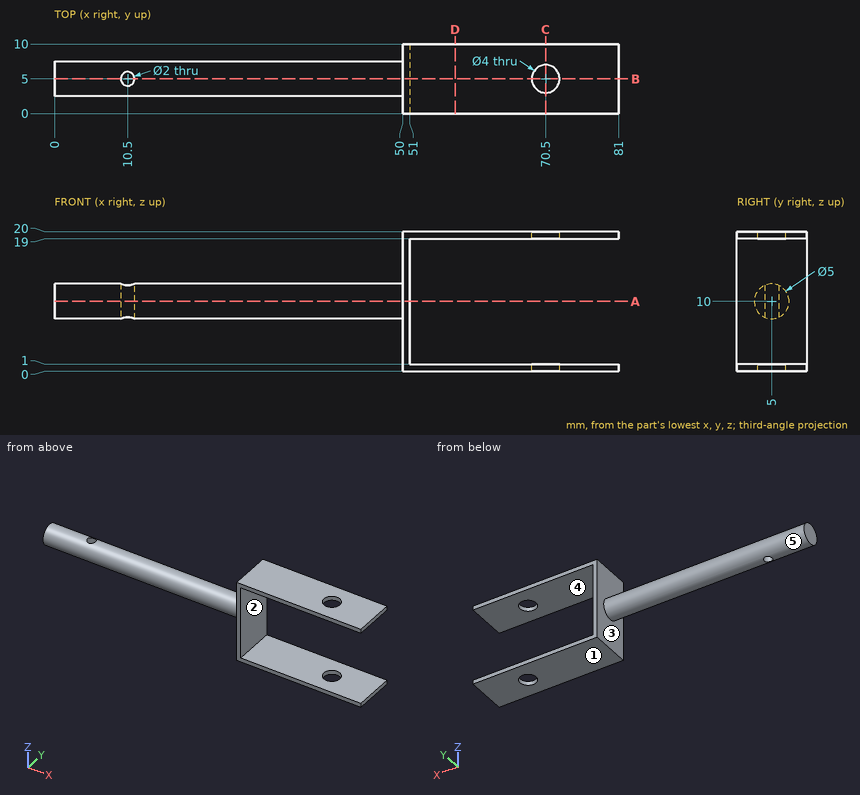
Input: dimensioned drawing with shaded views. Units: mm. Origin: part minimum x, y, z. A direction names the side the tool comes from. Give positions to 0.01 mm unless a question says otherwise; leave off trailing zeros. Order: outer loops, then holes, each group sorted by start corner. A loop starts at its lowest first (then second) coordinate and runs counter-clockwise, first axis right, second up. Notation, with made-up numbers: (55, 27.5) -> (98, 27.5) arc R25 cw to (98, 48.5) -> close; hole circle Ø9 at (-26, 39.25). An arc over 180 degrees is marked (long way). Answer as a JSON object with one key per item and string values.
Q1. First-contact query: pin 1 (1.6 mm diameter, centred on x = 10.5, y = 5, fed in from +Z); pin 2 (3 mm diameter, centred on x = 32.5, y = 6, fed in from +Z); pin 3 (1.5 mm diameter, centred on x = 44, y = 6, fed in from -Z); pin 4 (3 mm diameter, centred on y = 6.5, z = 12, fed in from +X). Flat tips, straight axial feed; report the tip coordinate or a pass-through.
Entries:
{"pin 1": "passes through", "pin 2": "stops at z = 12.5", "pin 3": "stops at z = 7.51", "pin 4": "stops at x = 51"}
Q2. Section D-D (x = 57.5). Output: boundary loops of the cut face in (y, z), plus the area to 3 significant figures.
Entries:
{"outline": "(0, 0) -> (10, 0) -> (10, 1) -> (0, 1) -> close; (0, 19) -> (10, 19) -> (10, 20) -> (0, 20) -> close", "area": "20.0 mm^2"}
Q3. Material intervals for probe 1 along X at (y, z) = (5, 8.6); probe 2 along X at (y, z) = (5, 19.75); probe 3 along Z at (x, y) = (69.5, 1.5), sorted ascending.
Entries:
{"probe 1": "x = 0 to 9.5, 11.5 to 51", "probe 2": "x = 50 to 68.5, 72.5 to 81", "probe 3": "z = 0 to 1, 19 to 20"}
Q4. Section A-A (z = 10). Output: boundary loops of the cut face in (x, y), plus the area to 3 significant figures.
Entries:
{"outline": "(0, 2.5) -> (50, 2.5) -> (50, 0) -> (51, 0) -> (51, 10) -> (50, 10) -> (50, 7.5) -> (0, 7.5) -> close; hole circle Ø2 at (10.5, 5)", "area": "257 mm^2"}
Q5. Access query for the marked faces 1, 2 and 3. Directions: +Z, -Z, +X, -X, +Y, -Y. A direction counts if a zero-diameter tool reaches every point of the face in a straight line with its end or side. Return the directions, or none.
Entries:
{"face 1": "-Z, +X, -X, +Y, -Y", "face 2": "+X, +Y, -Y", "face 3": "-X"}
Q6. Section B-B (y = 5). Output: boundary loops of the cut face in (x, z), plus the area to 3 significant figures.
Entries:
{"outline": "(0, 7.5) -> (9.5, 7.5) -> (9.5, 12.5) -> (0, 12.5) -> close; (11.5, 7.5) -> (50, 7.5) -> (50, 0) -> (68.5, 0) -> (68.5, 1) -> (51, 1) -> (51, 19) -> (68.5, 19) -> (68.5, 20) -> (50, 20) -> (50, 12.5) -> (11.5, 12.5) -> close; (72.5, 0) -> (81, 0) -> (81, 1) -> (72.5, 1) -> close; (72.5, 19) -> (81, 19) -> (81, 20) -> (72.5, 20) -> close", "area": "312 mm^2"}
Q7. Section C-C (x = 70.5). Output: boundary loops of the cut face in (y, z), plus the area to 3 significant figures.
Entries:
{"outline": "(0, 0) -> (3, 0) -> (3, 1) -> (0, 1) -> close; (0, 19) -> (3, 19) -> (3, 20) -> (0, 20) -> close; (7, 0) -> (10, 0) -> (10, 1) -> (7, 1) -> close; (7, 19) -> (10, 19) -> (10, 20) -> (7, 20) -> close", "area": "12.0 mm^2"}
Q8. Draft query along Y for the marked faces 4 and 5. Return one class per face: released by +Y, released by -Y, zero draft, split by the parting line, or undercut.
Entries:
{"face 4": "zero draft", "face 5": "split by the parting line"}
